Print and shaded views of the part. All mm, measured from the part's lowest x, y and z. A direction names the side the tool comes from. Round coordinates to 2 decimals unless told otherwise and drop trailing zeros. Loops run counter-clockwise (first coordinate to the right, second up) from the corner with the lowest first, then second, coordinate; pieces in that order, holes last. Notation, with made-up numbers: (46, 34) - (98, 34) arc R25 ccw to (98, 47) - close; hole circle Ø2 at (71.25, 32.25). An arc over 180 degrees is marked (long way). Answer as a JSON object with one key per item and string values.
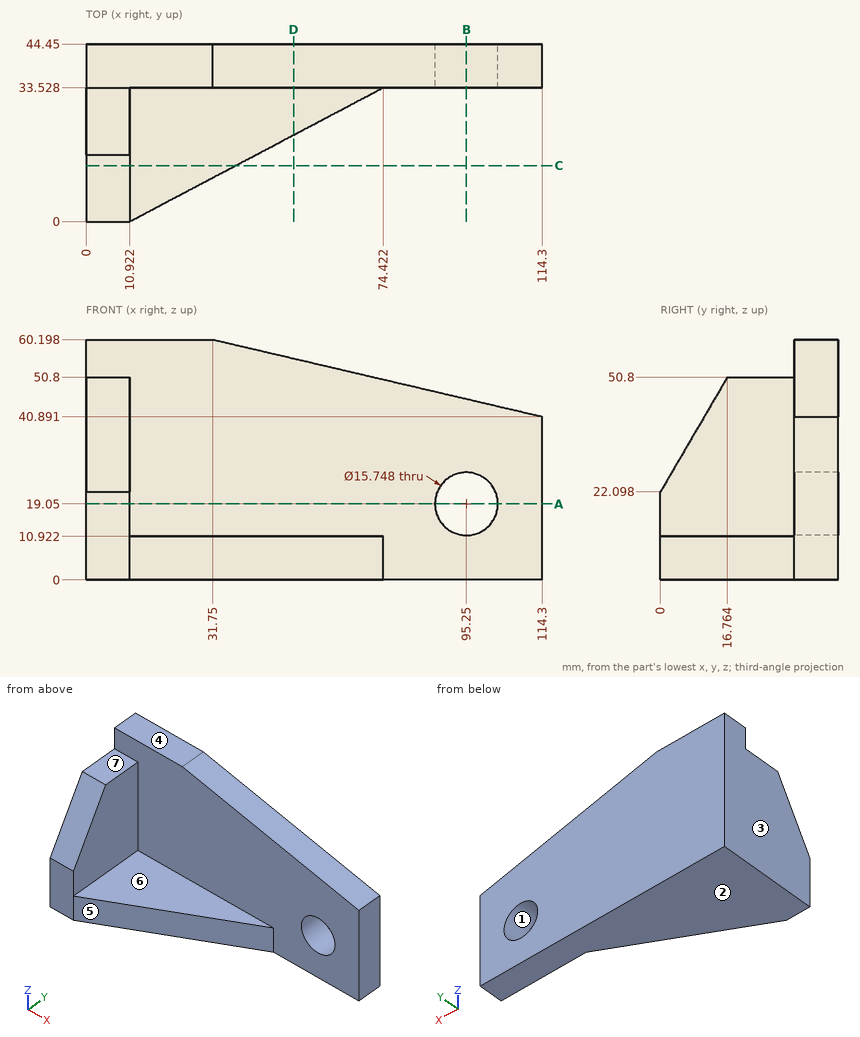
1) Slice it at A-A on z = 19.05. List the corners of the cut face in (x, y).
Values follow:
{"outline": "(0, 0) - (10.92, 0) - (10.92, 33.53) - (87.38, 33.53) - (87.38, 44.45) - (0, 44.45) - close; (103.12, 33.53) - (114.3, 33.53) - (114.3, 44.45) - (103.12, 44.45) - close"}
2) Slice it at C-C on y = 14. List the corners of the cut face in (x, z), then the cut area to 3 significant figures.
Values follow:
{"outline": "(0, 0) - (37.44, 0) - (37.44, 10.92) - (10.92, 10.92) - (10.92, 46.07) - (0, 46.07) - close", "area": "793 mm²"}
3) Probe probe 1 along X at (y, z) = (40, 19); probe 2 along Y at (x, z) = (56.5, 17); probe 3 along X at (y, z) = (13.5, 39.5). List the from-to ranges inside material, lowest first.
Values follow:
{"probe 1": "0 to 87.38, 103.12 to 114.3", "probe 2": "33.53 to 44.45", "probe 3": "0 to 10.92"}
4) Two-plate mould, pull along Z, no slides. Class the marked faces 1, 2, 3 and 4: pulls with the +Z half, pulls with the -Z half, needs draft (parallel to the pull), parting line crosses it, or undercut.
Values follow:
{"face 1": "undercut", "face 2": "pulls with the -Z half", "face 3": "needs draft", "face 4": "pulls with the +Z half"}
5) Tool access for the marked faces 5, 6 and 7: list every direction of +Z, -Z, +X, -X, +Y, -Y with a clear straight run to the whole face (end or side of a thin tool).
Values follow:
{"face 5": "+Z, -Z, +X, -Y", "face 6": "+Z, +X, -Y", "face 7": "+Z, +X, -X, -Y"}
6) Slice it at D-D on x = 52. List the corners of the cut face in (y, z).
Values follow:
{"outline": "(21.69, 0) - (44.45, 0) - (44.45, 55.46) - (33.53, 55.46) - (33.53, 10.92) - (21.69, 10.92) - close"}
7) Drop flat-ended pins along their axis: P1, Ø3, axis at y = 18.5, z = 19.5, coming from the +X side; P2, Ø17, axis at x = 28, y = 21, coming from the +Z side; P3, Ø12, axis at x = 63, z = 22.5, coming from the -Y side; P4, Ø6, axis at x = 36.5, y = 7.5, coming from the +Z side. Give the stop position or say it passes through.
Values follow:
{"P1": "x = 10.92", "P2": "z = 10.92", "P3": "y = 33.53", "P4": "through"}
8) Slice it at B-B on x = 95.25. List the corners of the cut face in (y, z), then the cut area to 3 significant figures.
Values follow:
{"outline": "(33.53, 0) - (44.45, 0) - (44.45, 11.18) - (33.53, 11.18) - close; (33.53, 26.92) - (44.45, 26.92) - (44.45, 45.35) - (33.53, 45.35) - close", "area": "323 mm²"}
